```python
from build123d import *

# Parameters (mm, degrees)
SKETCH1_W           = 23
SKETCH1_H           = 38
BOSS_EXTRUDE1_DEPTH = 4.87
FILLET1_R           = 1
SKETCH2_W           = 23
SKETCH2_H           = 38
SKETCH2_W_2         = 18.6
SKETCH2_H_2         = 33.6
CUT_EXTRUDE1_DEPTH  = 1
SKETCH3_W           = 5
SKETCH3_H           = 10
CUT_EXTRUDE2_DEPTH  = 4.37
CUT_EXTRUDE3_REACH  = 24.635
SKETCH4_W           = 2.5
SKETCH4_H           = 4.5
SKETCH5_R           = 2.5
BOSS_EXTRUDE2_DEPTH = 15.5
SKETCH6_R           = 0.95
CUT_EXTRUDE4_DEPTH  = 6
SKETCH7_W           = 3
SKETCH7_H           = 5
CUT_EXTRUDE5_DEPTH  = 4.2


with BuildPart() as part:
    # Sketch1 → Boss-Extrude1 (new body)
    with BuildSketch(Plane(origin=(0, 0, 0), x_dir=(1, 0, 0), z_dir=(0, 1, 0))):
        Rectangle(SKETCH1_W, SKETCH1_H)
    extrude(amount=BOSS_EXTRUDE1_DEPTH)

    # Fillet1
    fillet1_edges = [part.edges().sort_by_distance(p)[0] for p in [
        (0, 4.87, 19),
        (11.5, 4.87, 0),
        (0, 4.87, -19),
        (11.5, 2.435, 19),
        (11.5, 2.435, -19),
    ]]
    fillet(fillet1_edges, radius=FILLET1_R)

    # Sketch2 → Cut-Extrude1 (cut)
    with BuildSketch(Plane.XZ):
        Rectangle(SKETCH2_W, SKETCH2_H)
        Rectangle(SKETCH2_W_2, SKETCH2_H_2, mode=Mode.SUBTRACT)
    extrude(amount=-CUT_EXTRUDE1_DEPTH, mode=Mode.SUBTRACT)

    # Sketch3 → Cut-Extrude2 (cut)
    with BuildSketch(Plane.XZ):
        Rectangle(SKETCH3_W, SKETCH3_H)
    extrude(amount=-CUT_EXTRUDE2_DEPTH, mode=Mode.SUBTRACT)

    # Sketch4 → Cut-Extrude3 (cut, up to next)
    with BuildSketch(Plane.XZ.offset(-4.37), mode=Mode.PRIVATE) as cut_extrude3_sk1:
        Rectangle(SKETCH4_W, SKETCH4_H)
    cut_extrude3_tool1 = extrude(cut_extrude3_sk1.sketch, amount=-CUT_EXTRUDE3_REACH, mode=Mode.PRIVATE) & part.part
    add(cut_extrude3_tool1.solids().sort_by_distance((0, 4.37, 0))[0], mode=Mode.SUBTRACT)

    # Sketch5 → Boss-Extrude2 (add)
    with BuildSketch(Plane.XZ):
        with Locations(Location((0, -11, 0), (0, 0, 90))):
            Circle(SKETCH5_R)
        with Locations(Location((0, 11, 0), (0, 0, 90))):
            Circle(SKETCH5_R)
    extrude(amount=BOSS_EXTRUDE2_DEPTH)

    # Sketch6 → Cut-Extrude4 (cut)
    with BuildSketch(Plane.XZ.offset(15.5)):
        with Locations(Location((0, -11, 0), (0, 0, 270))):
            Circle(SKETCH6_R)
        with Locations(Location((0, 11, 0), (0, 0, 270))):
            Circle(SKETCH6_R)
    extrude(amount=-CUT_EXTRUDE4_DEPTH, mode=Mode.SUBTRACT)

    # Sketch7 → Cut-Extrude5 (cut)
    with BuildSketch(Plane(origin=(11.5, 0, 0), x_dir=(0, 0, -1), z_dir=(1, 0, 0))):
        Rectangle(SKETCH7_W, SKETCH7_H)
    extrude(amount=-CUT_EXTRUDE5_DEPTH, mode=Mode.SUBTRACT)


solid = part.part
```
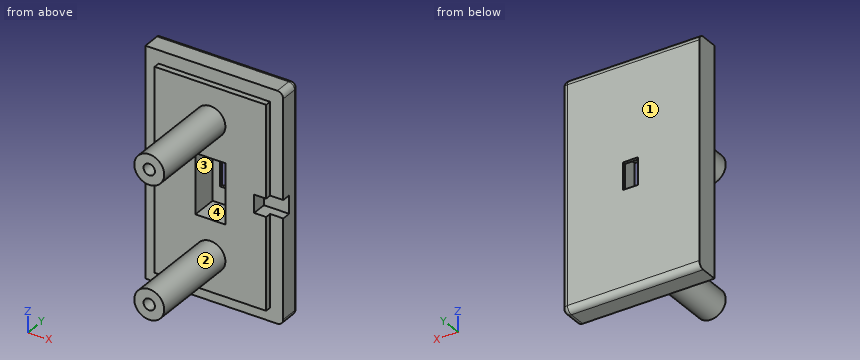
Read the model definition and answer for the solid it produces. Units are mm, in the model's axes. Face numbers are marked on the shaded views. Coordinates: 2 decimals unless noted, no trailing zeros. Order: outer loops, then holes, each group sorted by start corner. A loop starts at its lowest first (then second) coordinate and runs counter-clockwise, first axis right, second up. Notation, with made-up numbers: (21.25, 28) - (62.25, 28) arc R34 ccw to (62.25, 63) - close; hole circle Ø11 at (-8, -35.5). An arc over 180 degrees is marked (long way). Answer as a JSON object with one key per item and string values. Group by question number.
Item 1: Flat-ended cylindrical pins translate along their axes: P1, Ø0.8, axis at x = -4.5, y = 0.5, coming from the +Z side; P2, Ø0.6, axis at x = 0, z = -10.5, coming from the -Y side; P3, Ø3, axis at y = 0.5, z = -1, coming from the +X side; P4, Ø0.6, axis at x = 0, y = 4.5, coming from the +Z side. Find the tip coordinate at first contact, or state that the pin passes through.
Item 2: Section D-D (x = 7.75) is taken. Give the vertices of the cut face in (y, z).
Item 3: Section B-B (y = -12.25) is taken. Give the vertices of the cut face in (x, z).
Item 4: The mould has two halves that part along X. Classify the marked faces 1, 2, 3 and 4: +X half, -X half, draft (parallel to the pull), parting line (faces both ways), or undercut.
Item 5: Consider probe 1 along X at (y, z) = (-10.75, -11); probe 2 along Z at (x, y) = (-0.5, -11.25); probe 3 along X at (y, z) = (4, 15.5). Determine where each line is inside the solid, lowest interval first. Write a range as from..to.
Item 6: Section C-C (z = -11) is taken. Give the vertices of the cut face in (x, y), plus the area to 3 significant figures.
Results are:
{
 "1": {"P1": "stops at z = 16.8", "P2": "stops at y = -9.5", "P3": "stops at x = 11.5", "P4": "stops at z = 18.94"},
 "2": {"outline": "(0, -16.8) - (1, -16.8) - (1, -19) - (3.87, -19) arc R1 ccw to (4.87, -18) - (4.87, 18) arc R1 ccw to (3.87, 19) - (1, 19) - (1, 16.8) - (0, 16.8) - (0, 1.5) - (2.5, 1.5) - (2.5, -1.5) - (0, -1.5) - close"},
 "3": {"outline": "circle Ø5 at (0, -11); circle Ø5 at (0, 11); hole circle Ø1.9 at (0, -11); hole circle Ø1.9 at (0, 11)"},
 "4": {"face 1": "draft", "face 2": "parting line", "face 3": "undercut", "face 4": "undercut"},
 "5": {"probe 1": "x = -2.5..-0.95, 0.95..2.5", "probe 2": "z = -13.45..-11.81, -10.19..-8.55, 8.55..10.19, 11.81..13.45", "probe 3": "x = -11.5..11.49"},
 "6": {"outline": "(-11.5, 1) - (-9.3, 1) - (-9.3, 0) - (-2.5, 0) - (-2.5, -15.5) - (-0.95, -15.5) - (-0.95, -9.5) - (0.95, -9.5) - (0.95, -15.5) - (2.5, -15.5) - (2.5, 0) - (9.3, 0) - (9.3, 1) - (11.5, 1) - (11.5, 3.87) arc R1 ccw to (10.5, 4.87) - (-11.5, 4.87) - close", "area": "173 mm^2"}
}
